Part model, mm, in its own coordinate system. Coordinates: 2 decimals unless noted, no trailing zeros. Order: outer loops, then holes, each group sorted by start corner. A loop starts at its lowest first (then second) coordinate and runs counter-clockwise, first axis right, second up. Notation, with made-up numbers: (5, -35) - (50, -35) arc R25 cw to (50, -6) - close; hole circle Ø4 at (86, 34). An arc over 180 degrees is marked (long way). Use a Markdown table: item, result. Add a question column.
1) Wall check: L1, parallel to Y at x = 76, z = 3.25; L2, parallel to Y at x = 8.5, z = 1.05; L3, parallel to X at y = 87.5, z = 1.9. Give the ranges that are in metal, low to high. Write a range as [from, to].
2) Drop a flat-ended pin along its axis: P1, Ø1.6, axis at x = 134.5, y = 52.5, coming from the +Z side. Give the stop position or say it passes through.
3) Saw through at D-D on y = 35.5. Count the separate pieces of the cut face and the enclosed holes in it, then the cut area to 4 significant figures.
4) Saw through at A-A on y = 68.5. List the corners of the cut face in (x, z).
5) Saw through at B-B on x = 113. List the corners of the cut face in (y, z), then the cut area to 3 significant figures.
6) Saw through at C-C on x = 51. List the corners of the cut face in (y, z).
```python
from build123d import *

# Parameters (mm, degrees)
SKETCH006_W     = 143
SKETCH006_H     = 96
PAD003_DEPTH    = 3.5
SKETCH007_W     = 68
SKETCH007_H     = 30
POCKET003_DEPTH = 3.501
SKETCH008_W     = 11
SKETCH008_H     = 9
POCKET004_DEPTH = 3.501
SKETCH009_W     = 51
SKETCH009_H     = 5
POCKET005_DEPTH = 3.501
SKETCH010_R     = 1
POCKET006_DEPTH = 3.501


with BuildPart() as part:
    # Sketch006 → Pad003 (new body)
    with BuildSketch(Plane.XY):
        with Locations((71.5, 48)):
            Rectangle(SKETCH006_W, SKETCH006_H)
    extrude(amount=PAD003_DEPTH)

    # Sketch007 (on Face6 of Pad003) → Pocket003 (cut, through all)
    with BuildSketch(Plane.XY.offset(3.5)):
        with Locations((45.5, 68)):
            Rectangle(SKETCH007_W, SKETCH007_H)
    extrude(amount=-POCKET003_DEPTH, mode=Mode.SUBTRACT)

    # Sketch008 (on Face5 of Pocket003) → Pocket004 (cut, through all)
    with BuildSketch(Plane.XY.offset(3.5)):
        with Locations((17.5, 42.5)):
            Rectangle(SKETCH008_W, SKETCH008_H)
        with Locations((29.5, 42.5)):
            Rectangle(SKETCH008_W, SKETCH008_H)
        with Locations((41.5, 42.5)):
            Rectangle(SKETCH008_W, SKETCH008_H)
        with Locations((53.5, 42.5)):
            Rectangle(SKETCH008_W, SKETCH008_H)
        with Locations((65.5, 42.5)):
            Rectangle(SKETCH008_W, SKETCH008_H)
        with Locations((77.5, 42.5)):
            Rectangle(SKETCH008_W, SKETCH008_H)
        with Locations((89.5, 42.5)):
            Rectangle(SKETCH008_W, SKETCH008_H)
        with Locations((101.5, 42.5)):
            Rectangle(SKETCH008_W, SKETCH008_H)
        with Locations((113.5, 42.5)):
            Rectangle(SKETCH008_W, SKETCH008_H)
        with Locations((125.5, 42.5)):
            Rectangle(SKETCH008_W, SKETCH008_H)
        with Locations((17.5, 32.5)):
            Rectangle(SKETCH008_W, SKETCH008_H)
        with Locations((29.5, 32.5)):
            Rectangle(SKETCH008_W, SKETCH008_H)
        with Locations((41.5, 32.5)):
            Rectangle(SKETCH008_W, SKETCH008_H)
        with Locations((53.5, 32.5)):
            Rectangle(SKETCH008_W, SKETCH008_H)
        with Locations((65.5, 32.5)):
            Rectangle(SKETCH008_W, SKETCH008_H)
        with Locations((77.5, 32.5)):
            Rectangle(SKETCH008_W, SKETCH008_H)
        with Locations((89.5, 32.5)):
            Rectangle(SKETCH008_W, SKETCH008_H)
        with Locations((101.5, 32.5)):
            Rectangle(SKETCH008_W, SKETCH008_H)
        with Locations((113.5, 32.5)):
            Rectangle(SKETCH008_W, SKETCH008_H)
        with Locations((125.5, 32.5)):
            Rectangle(SKETCH008_W, SKETCH008_H)
        with Locations((17.5, 22.5)):
            Rectangle(SKETCH008_W, SKETCH008_H)
        with Locations((29.5, 22.5)):
            Rectangle(SKETCH008_W, SKETCH008_H)
        with Locations((41.5, 22.5)):
            Rectangle(SKETCH008_W, SKETCH008_H)
        with Locations((53.5, 22.5)):
            Rectangle(SKETCH008_W, SKETCH008_H)
        with Locations((65.5, 22.5)):
            Rectangle(SKETCH008_W, SKETCH008_H)
        with Locations((77.5, 22.5)):
            Rectangle(SKETCH008_W, SKETCH008_H)
        with Locations((89.5, 22.5)):
            Rectangle(SKETCH008_W, SKETCH008_H)
        with Locations((101.5, 22.5)):
            Rectangle(SKETCH008_W, SKETCH008_H)
        with Locations((113.5, 22.5)):
            Rectangle(SKETCH008_W, SKETCH008_H)
        with Locations((125.5, 22.5)):
            Rectangle(SKETCH008_W, SKETCH008_H)
        with Locations((17.5, 12.5)):
            Rectangle(SKETCH008_W, SKETCH008_H)
        with Locations((29.5, 12.5)):
            Rectangle(SKETCH008_W, SKETCH008_H)
        with Locations((41.5, 12.5)):
            Rectangle(SKETCH008_W, SKETCH008_H)
        with Locations((53.5, 12.5)):
            Rectangle(SKETCH008_W, SKETCH008_H)
        with Locations((65.5, 12.5)):
            Rectangle(SKETCH008_W, SKETCH008_H)
        with Locations((77.5, 12.5)):
            Rectangle(SKETCH008_W, SKETCH008_H)
        with Locations((89.5, 12.5)):
            Rectangle(SKETCH008_W, SKETCH008_H)
        with Locations((101.5, 12.5)):
            Rectangle(SKETCH008_W, SKETCH008_H)
        with Locations((113.5, 12.5)):
            Rectangle(SKETCH008_W, SKETCH008_H)
        with Locations((125.5, 12.5)):
            Rectangle(SKETCH008_W, SKETCH008_H)
    extrude(amount=-POCKET004_DEPTH, mode=Mode.SUBTRACT)

    # Sketch009 (on Face5 of Pocket004) → Pocket005 (cut, through all)
    with BuildSketch(Plane.XY.offset(3.5)):
        with Locations((110.5, 79.28)):
            Rectangle(SKETCH009_W, SKETCH009_H)
        with Locations((110.5, 61.5)):
            Rectangle(SKETCH009_W, SKETCH009_H)
    extrude(amount=-POCKET005_DEPTH, mode=Mode.SUBTRACT)

    # Sketch010 (on Face5 of Pocket005) → Pocket006 (cut, through all)
    with BuildSketch(Plane.XY.offset(3.5)):
        with Locations((8.5, 87.5)):
            Circle(SKETCH010_R)
        with Locations((134.5, 87.5)):
            Circle(SKETCH010_R)
        with Locations((8.5, 52.5)):
            Circle(SKETCH010_R)
        with Locations((134.5, 52.5)):
            Circle(SKETCH010_R)
        with Locations((8.5, 8.5)):
            Circle(SKETCH010_R)
        with Locations((134.5, 8.5)):
            Circle(SKETCH010_R)
    extrude(amount=-POCKET006_DEPTH, mode=Mode.SUBTRACT)


solid = part.part
```
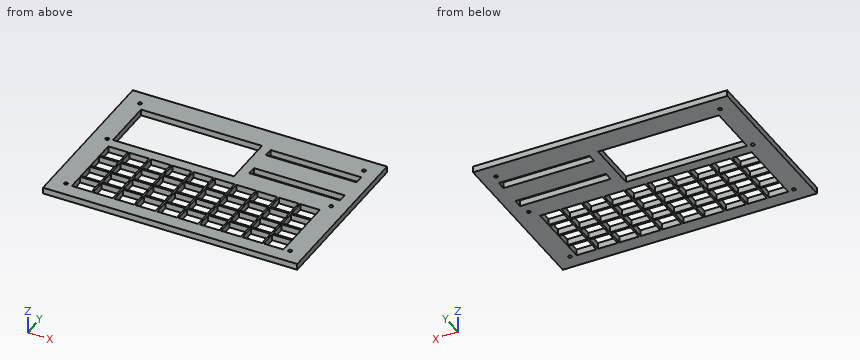
Results are:
| question | item | result |
|---|---|---|
| 1 | L1 | [0, 8], [17, 18], [27, 28], [37, 38], [47, 53], [83, 96] |
| 1 | L2 | [0, 7.5], [9.5, 51.5], [53.5, 86.5], [88.5, 96] |
| 1 | L3 | [0, 7.5], [9.5, 133.5], [135.5, 143] |
| 2 | P1 | through |
| 3 | separate pieces | 11 |
| 3 | enclosed holes | 0 |
| 3 | area | 115.5 mm2 |
| 4 | outline | (0, 0) - (11.5, 0) - (11.5, 3.5) - (0, 3.5) - close; (79.5, 0) - (143, 0) - (143, 3.5) - (79.5, 3.5) - close |
| 5 | outline | (0, 0) - (8, 0) - (8, 3.5) - (0, 3.5) - close; (17, 0) - (18, 0) - (18, 3.5) - (17, 3.5) - close; (27, 0) - (28, 0) - (28, 3.5) - (27, 3.5) - close; (37, 0) - (38, 0) - (38, 3.5) - (37, 3.5) - close; (47, 0) - (59, 0) - (59, 3.5) - (47, 3.5) - close; (64, 0) - (76.78, 0) - (76.78, 3.5) - (64, 3.5) - close; (81.78, 0) - (96, 0) - (96, 3.5) - (81.78, 3.5) - close |
| 5 | area | 175 mm2 |
| 6 | outline | (0, 0) - (8, 0) - (8, 3.5) - (0, 3.5) - close; (17, 0) - (18, 0) - (18, 3.5) - (17, 3.5) - close; (27, 0) - (28, 0) - (28, 3.5) - (27, 3.5) - close; (37, 0) - (38, 0) - (38, 3.5) - (37, 3.5) - close; (47, 0) - (53, 0) - (53, 3.5) - (47, 3.5) - close; (83, 0) - (96, 0) - (96, 3.5) - (83, 3.5) - close |
